```python
from build123d import *

# Parameters (mm, degrees)
F0_R     = 2.65
F0_R_2   = 1.95
F1_DEPTH = 10
F2_R     = 2.65
F3_DEPTH = 10
F4_SIZE  = 1
F6_DEPTH = 2.7778161572
F7_DEPTH = 2.5241839428


with BuildPart() as f1:
    # F0 (on Top) → F1 (new body)
    with BuildSketch(Plane.XY):
        with Locations((0, 0.1268161572)):
            Circle(F0_R)
        with Locations((0, 0.1268161572)):
            Circle(F0_R_2, mode=Mode.SUBTRACT)
    extrude(amount=F1_DEPTH)

    # F2 (on face) → F3 (join)
    with BuildSketch(Plane.XY.offset(10)):
        with Locations((0, 0.1268161572)):
            Circle(F2_R)
    extrude(amount=F3_DEPTH)

    # F4
    f4_edges = [f1.edges().sort_by_distance(p)[0] for p in [
        (-2.65, 0.126816, 20),
    ]]
    chamfer(f4_edges, length=F4_SIZE)

    # F5 (on Front) → F6 (cut, through all)
    with BuildSketch(Plane.XZ):
        with BuildLine():
            Line((-0.8353080657, 13.1434470012), (-0.8353080657, 12.2838566395))
            Line((-0.8353080657, 12.2838566395), (0.9646919343, 12.2838566395))
            Line((0.9646919343, 12.2838566395), (0.9646919343, 12.9951966612))
            ThreePointArc((0.9646919343, 12.9951966612), (0.0983848931, 13.4784090943), (-0.8353080657, 13.1434470012))
        make_face()
        with BuildLine():
            Line((0.9646919343, 12.2838566395), (-0.8353080657, 12.2838566395))
            Line((-0.8353080657, 12.2838566395), (-0.8353080657, 13.1434470012))
            ThreePointArc((-0.8353080657, 13.1434470012), (-0.4666032996, 11.1798111171), (1.1985971611, 12.2838566395))
            ThreePointArc((1.1985971611, 12.2838566395), (1.1386202546, 12.6582615946), (0.9646919343, 12.9951966612))
            Line((0.9646919343, 12.9951966612), (0.9646919343, 12.2838566395))
        make_face()
        with BuildLine():
            Line((-0.8353080657, 20.0238556888), (-0.8353080657, 13.1434470012))
            ThreePointArc((-0.8353080657, 13.1434470012), (0.0983848931, 13.4784090943), (0.9646919343, 12.9951966612))
            Line((0.9646919343, 12.9951966612), (0.9646919343, 20.0238556888))
            Line((0.9646919343, 20.0238556888), (-0.8353080657, 20.0238556888))
        make_face()
    extrude(amount=-F6_DEPTH, mode=Mode.SUBTRACT)

    # F7 (cut, through all): a face of the model
    f7_faces = [f1.faces().sort_by_distance(p)[0] for p in [
        (0.0489712617, 0, 15.4729630627),
    ]]
    extrude(f7_faces, amount=-F7_DEPTH, mode=Mode.SUBTRACT)


solid = f1.part
```
Read the model definition and answer for the solid it produces. Units are mm, in the model's axes. A direction names the side the tool comes from. Round coordinates to 2 decimals unless told otherwise and drop trailing zeros. Write each loop counter-clockwise with the first axis right and the second up, starting at its lowest first coordinate (ties: lowest second). Pieces come first, ordered by that corner, then holes. Notation, with made-up numbers: (-6.5, 89.25) -> (51.5, 89.25) arc R24 ccw to (51.5, 108.25) -> close; hole circle Ø5 at (86, 63.25). An arc over 180 degrees is marked (long way). Answer in a Markdown table with one row per item. Add a question column.
1) Determine the mould class of faces 1 (the face through (0, 0, 10)), 2 (the face through (-1, 2, 0)), 3 (the face through (-1.547, -1.06, 4.93)), 4 (the face through (-1.92, 0.16, 19.73)) for opening direction X: pulls with the +X half, pulls with the -X half, needs draft (parallel to the pull), parting line crosses it, or undercut.
2) Find section C-C, the plane z = 3.5. Determine the outline of the cut face in (x, y), and give its area (3 significant figures).
3) Consider line 1 (Y direction, x = 0, z = 4.5); line 2 (X direction, y = -0.7, z = 18.5); line 3 (Z direction, x = 0, y = 0.85). Determine where each line is inside the solid, lowest interval first.
4) Which of the six approach directions +Z, -Z, +X, -X, +Y, -Y give full straight-line access (tool end or side, diameter ignored) to faces 5 (the face through (-0.835, 0, 17)), 6 (the face through (2.53, 0.92, 9.37))?
5) Find section A-A, the plane x = 0. Determine the outline of the cut face in (y, z), and give its area (3 significant figures).
6) Given P1, Ø1.2, axis at x = 1, y = 0.5, coming from the -Z side; P2, Ø1.5, axis at y = 1.5, z = 17, coming from the -X side; P3, Ø1.3, axis at y = 2, z = 17, coming from the -X side, each flat-ended and moving along its own axis, determine where each tip first touches the part or whether it passes through.
7) Find section B-B, the plane z = 13.5. Determine the outline of the cut face in (x, y), and give its area (3 significant figures).
Findings below:
| question | item | result |
|---|---|---|
| 1 | face 1 | undercut |
| 1 | face 2 | needs draft |
| 1 | face 3 | undercut |
| 1 | face 4 | pulls with the -X half |
| 2 | outline | circle Ø5.3 at (0, 0.13); hole circle Ø3.9 at (0, 0.13) |
| 2 | area | 10.1 mm² |
| 3 | line 1 | -2.52 to -1.82, 2.08 to 2.78 |
| 3 | line 2 | -2.52 to -0.84, 0.96 to 2.52 |
| 3 | line 3 | 10 to 11.09 |
| 4 | face 5 | +Z, +Y, -Y |
| 4 | face 6 | +Z, -Z |
| 5 | outline | (-2.52, 0) -> (-1.82, 0) -> (-1.82, 10) -> (2.08, 10) -> (2.08, 0) -> (2.78, 0) -> (2.78, 11.09) -> (-2.52, 11.09) -> close |
| 5 | area | 19.8 mm² |
| 6 | P1 | z = 10 |
| 6 | P2 | x = -2.58 |
| 6 | P3 | x = -2.35 |
| 7 | outline | (-0.84, -2.39) -> (-0.84, 2.64) arc R2.65 ccw to start; (0.96, -2.34) arc R2.65 ccw to (0.96, 2.59) -> close |
| 7 | area | 12.7 mm² |
